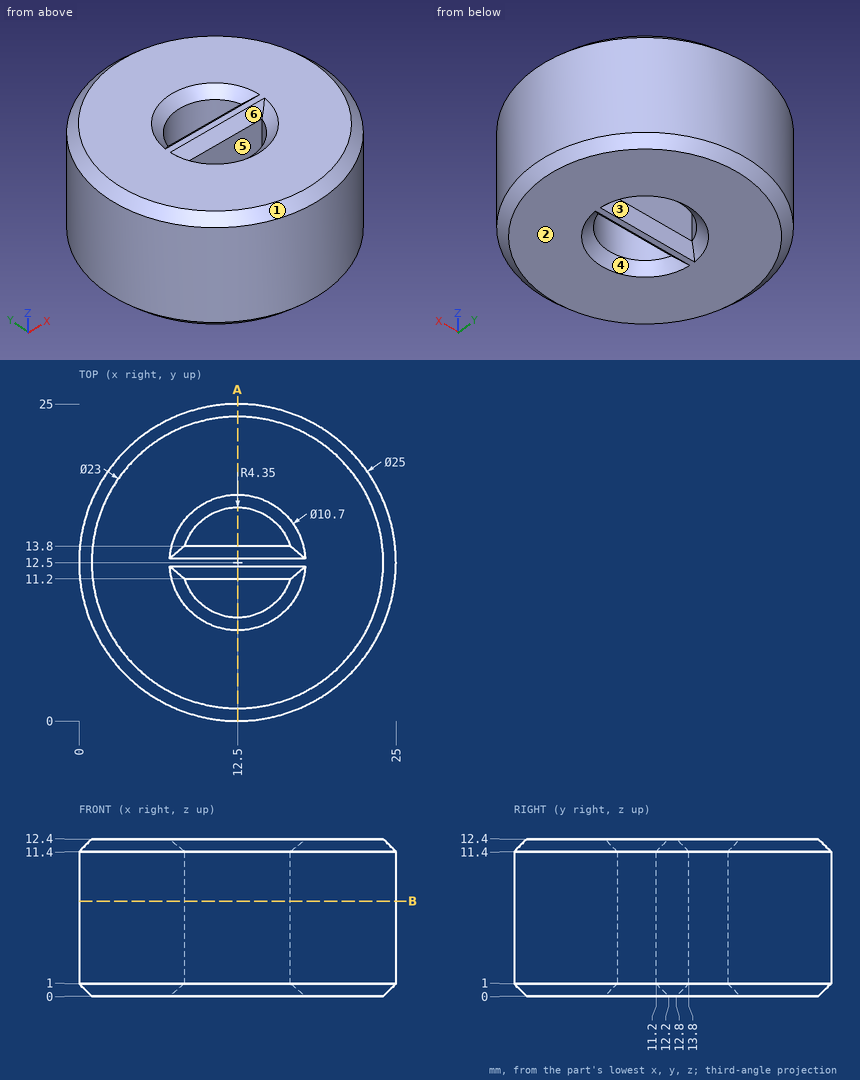
Check sheet for the drawn part. Datum: minimum x, y, z corner. Units: mm. A direction names the side the tool comes from. Round coordinates to 2 decimals unless told otherwise and drop trailing zeros. Loops run counter-clockwise (first coordinate to the right, second up) from the corner with the lowest first, then second, coordinate; pieces in that order, holes last. Notation, with made-up numbers: (72.5, 5) - (87.5, 5) arc R25 cw to (87.5, 29) - close; hole circle Ø11 at (71.25, -26). An arc over 180 degrees is marked (long way). Write item = value, one per line. Start each with the question number.
1. Section check A-A on x = 12.5. Enter the section's corners in (y, z).
2. Depth check by flat-ended pin: pin 1 (1.5 mm diameter, centred on y = 16.5, z = 6, fed in from -X); pin 2 (1 mm diameter, centred on x = 22, z = 9, fed in from -Y); pin 3 (2 mm diameter, centred on y = 17, z = 6, fed in from -X). Enter the tip coordinate at first touch or a pass-through.
3. Mould release check, pull along Y, two halves, no side actions. Record for the marked faces 1, 2 and 3: released by +Y, released by -Y, zero draft, split by the parting line, or undercut.
4. Set-up check for the marked faces 4, 5 and 6: record each of +Z, -Z, +X, -X, +Y, -Y from which the full face is reachable in a straight line by a thin tool's end or side.
5. Thickness scan on line 1 (Y direction, x = 12.5, z = 11.25); line 2 (Y direction, x = 16.5, z = 5.25); line 3 (X direction, y = 10.25, z = 2.5). Record the ranges inside material, lowest first.
6. Section check B-B on z = 7.5. Enter the section's corners in (x, y), then the cut area to 3 significant figures.
Working result:
q1.outline = (0, 1) - (1, 0) - (7.15, 0) - (8.15, 1) - (8.15, 11.4) - (7.15, 12.4) - (1, 12.4) - (0, 11.4) - close; (11.2, 1) - (12.2, 0) - (12.8, 0) - (13.8, 1) - (13.8, 11.4) - (12.8, 12.4) - (12.2, 12.4) - (11.2, 11.4) - close; (16.85, 1) - (17.85, 0) - (24, 0) - (25, 1) - (25, 11.4) - (24, 12.4) - (17.85, 12.4) - (16.85, 11.4) - close
q2.pin_1 = 0.43
q2.pin_2 = 3.83
q2.pin_3 = 0.5
q3.face_1 = split by the parting line
q3.face_2 = zero draft
q3.face_3 = undercut
q4.face_4 = -Z
q4.face_5 = +Z, -Z
q4.face_6 = +Z
q5.line_1 = 0 to 8.15, 11.2 to 13.8, 16.85 to 25
q5.line_2 = 0.66 to 10.79, 11.2 to 13.8, 14.21 to 24.34
q5.line_3 = 0.2 to 8.78, 16.22 to 24.8
q6.outline = circle Ø25 at (12.5, 12.5); hole (8.35, 11.2) arc R4.35 ccw to (16.65, 11.2) - close; hole (8.35, 13.8) - (16.65, 13.8) arc R4.35 ccw to start
q6.area = 454 mm^2
